Answer from the drawing. Dimensions are ordinates in mm from the lowest x, y and z of the part. Coordinates: 2 decimals unless noted, no trailing zeros. Loops run counter-clockwise (first coordinate to the right, second up) from the corner with the lowest first, then second, coordinate; pieces in that order, holes last. Notation, with made-up numbers: (5, 24.5) - (47, 24.5) arc R17 ccw to (47, 57.5) - close; hole circle Ø4 at (-9, 63). An arc over 180 degrees is marked (long way). Write each question's results on one line, items separated by ' | '. Start each with the question number.
1. Determine the mould class of the marked faces 1, 2 and 3 for opening direction Y: released by +Y, released by -Y, zero draft, split by the parting line, or undercut.
2. A cutting plane is placed at A-A on x = 7.55. Determine the outline of the cut face in (y, z).
3. A cutting plane is placed at C-C on z = 3. Determine the outline of the cut face in (x, y), then the cut area to 3 significant figures.
4. Find the intervals of material crossed by line 1 along Y through (x, z) = (7.55, 1); line 2 along Z through (x, y) = (6.25, 23.5); line 3 along Y through (x, z) = (1.5, 4.25), in increasing order. Write a range as [from, to].
5. A cutting plane is placed at B-B on y = 21.9. Determine the outline of the cut face in (x, z).
6. Each of these flat-tipped pins is pushed along its axis until it touches: P1, Ø4, axis at y = 22.5, z = 6, coming from the -X side; P2, Ø5.5, axis at x = 10, y = 23.5, coming from the +Z side; P3, Ø3, axis at x = 5.5, z = 3.5, coming from the +Y side. Where does it stop, or does it pass through?
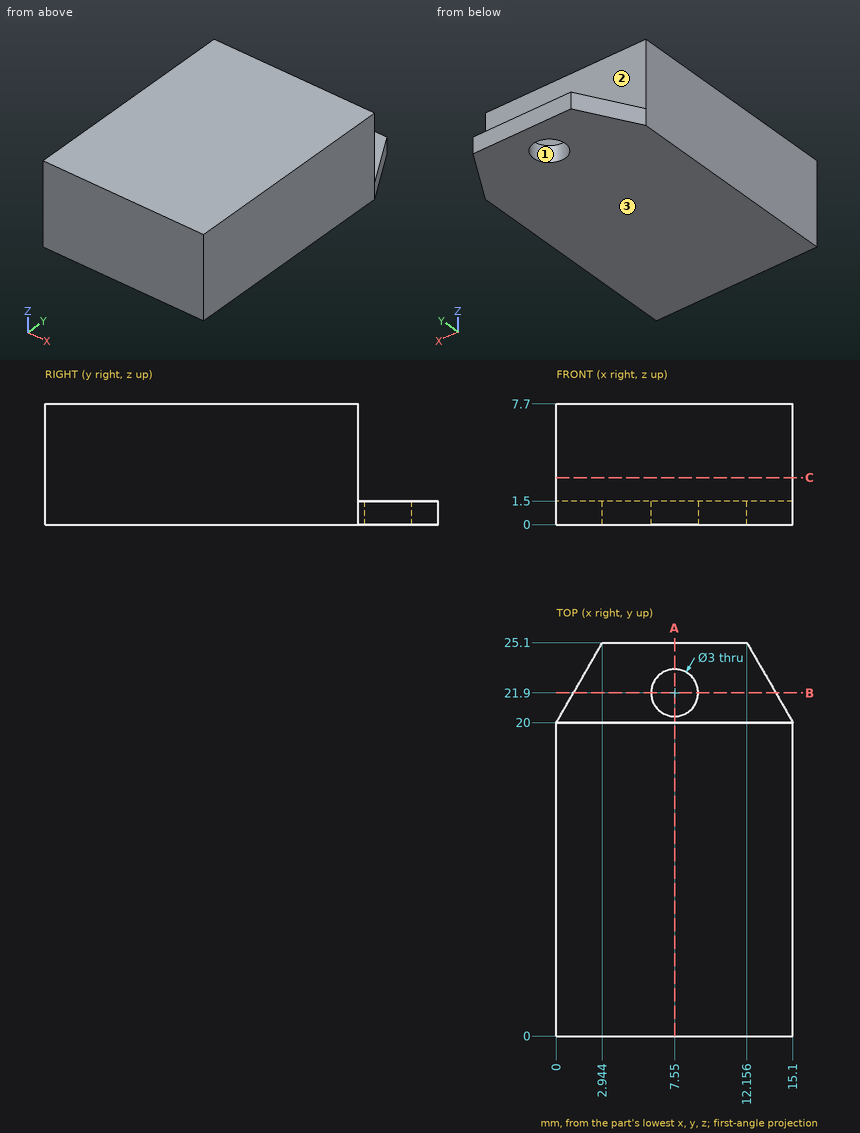
Values:
1) face 1: undercut | face 2: released by +Y | face 3: zero draft
2) outline: (0, 0) - (20.4, 0) - (20.4, 1.5) - (20, 1.5) - (20, 7.7) - (0, 7.7) - close; (23.4, 0) - (25.1, 0) - (25.1, 1.5) - (23.4, 1.5) - close
3) outline: (0, 0) - (15.1, 0) - (15.1, 20) - (0, 20) - close | area: 302 mm^2
4) line 1: [0, 20.4], [23.4, 25.1] | line 2: [0, 1.5] | line 3: [0, 20]
5) outline: (1.1, 0) - (6.05, 0) - (6.05, 1.5) - (1.1, 1.5) - close; (9.05, 0) - (14, 0) - (14, 1.5) - (9.05, 1.5) - close
6) P1: through | P2: z = 1.5 | P3: y = 20
